CAD build for the part. Positions are in the model's coordinates, mm. A direction names the side the tool comes from. Round coordinates to 2 decimals unless told otherwise and drop trailing zeros. One line per question, with ' | ' between items.
```python
from build123d import *

# Parameters (mm, degrees)
BOSS_EXTRUDE1_DEPTH = 19
CUT_EXTRUDE1_DEPTH  = 5
SKETCH5_R           = 5.5
CUT_EXTRUDE2_DEPTH  = 1
SKETCH6_W           = 3.836976741
SKETCH6_H           = 19
BOSS_EXTRUDE2_DEPTH = 6.17281
CUT_EXTRUDE3_DEPTH  = 19
SKETCH8_R           = 15.326273961
SKETCH8_R_2         = 13.53815969
CUT_EXTRUDE4_DEPTH  = 20
CUT_EXTRUDE5_START  = -20
SKETCH9_R           = 15.315451293
SKETCH9_R_2         = 13.53815969
CUT_EXTRUDE5_DEPTH  = 20


with BuildPart() as part:
    # Sketch1 → Boss-Extrude1 (new body)
    with BuildSketch(Plane.XY):
        with BuildLine():
            Line((9.418070486, 0.286487124), (9.423467442, 1.490329505))
            Line((9.423467442, 1.490329505), (13.272942596, 1.490329505))
            Line((13.272942596, 1.490329505), (13.272942596, -7.663136981))
            Line((13.272942596, -7.663136981), (0, -15.326273961))
            Line((0, -15.326273961), (-13.272942596, -7.663136981))
            Line((-13.272942596, -7.663136981), (-13.272942596, 0))
            Line((-13.272942596, 0), (-10.981676699, 1.490329505))
            Line((-10.981676699, 1.490329505), (-9.423467442, 1.490329505))
            Line((-9.423467442, 1.490329505), (-9.418070486, 0.286487124))
            Line((-9.418070486, 0.286487124), (-9.42470631, -1.19369635))
            ThreePointArc((-9.42470631, -1.19369635), (-0.052384082, -9.499855573), (9.41096903, -1.297559989))
            Line((9.41096903, -1.297559989), (9.418070486, 0.286487124))
        make_face()
    extrude(amount=BOSS_EXTRUDE1_DEPTH)

    # Sketch2 → Loft1 section 0
    with BuildSketch(Plane.XY.offset(19)):
        with BuildLine():
            Line((0, -15.326273961), (13.272942596, -7.663136981))
            Line((13.272942596, -7.663136981), (13.272942596, 7.663136981))
            Line((13.272942596, 7.663136981), (0, 15.326273961))
            Line((0, 15.326273961), (-13.272942596, 7.663136981))
            Line((-13.272942596, 7.663136981), (-13.272942596, -7.663136981))
            Line((-13.272942596, -7.663136981), (0, -15.326273961))
        make_face()
    # Sketch3 → Loft1 section 1
    with BuildSketch(Plane.XY.offset(24)):
        with BuildLine():
            Line((0, -9.814954576), (8.5, -4.907477288))
            Line((8.5, -4.907477288), (8.5, 4.907477288))
            Line((8.5, 4.907477288), (0, 9.814954576))
            Line((0, 9.814954576), (-8.5, 4.907477288))
            Line((-8.5, 4.907477288), (-8.5, -4.907477288))
            Line((-8.5, -4.907477288), (0, -9.814954576))
        make_face()
    loft()

    # Sketch4 → Cut-Extrude1 (cut)
    with BuildSketch(Plane.XY.offset(24)):
        Polygon((-8.5, 4.907477288), (-8.5, 10.418796673), (0, 15.326273961), (8.5, 10.418796673), (8.5, 4.907477288), align=None)
    extrude(amount=-CUT_EXTRUDE1_DEPTH, mode=Mode.SUBTRACT)

    # Sketch5 → Cut-Extrude2 (cut)
    with BuildSketch(Plane(origin=(0, 0, 19), x_dir=(-1, 0, 0), z_dir=(0, 0, -1))):
        with Locations((5.762922136, -0.004092629)):
            Circle(SKETCH5_R)
    extrude(amount=-CUT_EXTRUDE2_DEPTH, mode=Mode.SUBTRACT)

    # Sketch6 → Boss-Extrude2 (add)
    with BuildSketch(Plane(origin=(0, 1.490329505, 0), x_dir=(1, 0, 0), z_dir=(0, 1, 0))):
        with Locations((11.341955813, -9.5)):
            Rectangle(SKETCH6_W, SKETCH6_H)
    extrude(amount=BOSS_EXTRUDE2_DEPTH)

    # Sketch7 → Cut-Extrude3 (cut)
    with BuildSketch(Plane(origin=(0, 0, 0), x_dir=(-1, 0, 0), z_dir=(0, 0, -1))):
        with BuildLine():
            Line((13.53815969, 0), (15.326273961, 0))
            ThreePointArc((15.326273961, 0), (0, -15.326273961), (-15.326273961, 0))
            Line((-15.326273961, 0), (-13.53815969, 0))
            ThreePointArc((-13.53815969, 0), (0, -13.53815969), (13.53815969, 0))
        make_face()
    extrude(amount=-CUT_EXTRUDE3_DEPTH, mode=Mode.SUBTRACT)

    # Sketch8 → Cut-Extrude4 (cut)
    with BuildSketch(Plane(origin=(0, 0, 19), x_dir=(-1, 0, 0), z_dir=(0, 0, -1))):
        Circle(SKETCH8_R)
        Circle(SKETCH8_R_2, mode=Mode.SUBTRACT)
    extrude(amount=-CUT_EXTRUDE4_DEPTH, mode=Mode.SUBTRACT)

    # Sketch9 → Cut-Extrude5 (cut)
    with BuildSketch(Plane.XY.offset(19).offset(CUT_EXTRUDE5_START)):
        Circle(SKETCH9_R)
        Circle(SKETCH9_R_2, mode=Mode.SUBTRACT)
    extrude(amount=CUT_EXTRUDE5_DEPTH, mode=Mode.SUBTRACT)


with BuildPart() as cut_extrude5_kept_piece:
    # of the separate pieces the step leaves, the one the design keeps (cut_extrude5_pieces_kept)
    add(part.part.solids().sort_by_distance((9.41096903, -1.297559989, 0))[0])


solid = cut_extrude5_kept_piece.part
```
(1) Tool access for faces 1 (the face through (-0.244, -9.497, 9.367)), 2 (the face through (10, 7.663, 9)), 3 (the face through (-8.5, 6, 20)): list every direction of +Z, -Z, +X, -X, +Y, -Y with a clear straight run to the whole face (end or side of a thin tool).
Results found:
face 1: -Z, +Y | face 2: -Z, +X, -X, +Y | face 3: +Z, -Z, +Y
(2) Two-plate mould, pull along X, no slides. Class faces 4 (the face through (-6, 0, 20)), 5 (the face through (-11.755, 6.716, 19.439)), 6 (the face through (0.06, -13.54, 10.17)): released by +X, released by -X, zero draft, split by the parting line, or undercut.
Results found:
face 4: undercut | face 5: released by -X | face 6: split by the parting line
(3) Drop flat-ended pins along their axis: P1, Ø12, axis at x = 1, y = 6.5, coming from the -Z side; P2, Ø1, axis at x = 10, y = -0.5, coming from the +Z side; P3, Ø2.5, axis at x = -9, y = -1.5, coming from the +Z side; P4, Ø0.5, axis at x = -10, z = 11.5, coming from the +Y side. Give the stop position or say it passes through.
Results found:
P1: stops at z = 19 | P2: stops at z = 22.95 | P3: stops at z = 24 | P4: stops at y = 1.49
(4) Probe L1, parallel to Y at x = -8, z = 21; L2, parallel to Z at x = -5.5, y = -6.5; L3, parallel to Z at x = -3, y = 3.75. List the from-to ranges inside material, lowest first.
Results found:
L1: y = -8.5 to 4.91 | L2: z = 19 to 24 | L3: z = 20 to 24
